```python
from build123d import *

# Parameters (mm, degrees)
SKETCH_W     = 6
SKETCH_H     = 20
PAD_DEPTH    = 4
PAD001_DEPTH = 7
SKETCH002_W  = 2.5
SKETCH002_H  = 20
PAD002_DEPTH = 7
SKETCH003_W  = 4
SKETCH003_H  = 7.068021
PAD003_DEPTH = 9
PAD004_DEPTH = 4
FILLET_R     = 1
FILLET001_R  = 1


with BuildPart() as part:
    # Sketch → Pad (new body)
    with BuildSketch(Plane.XY):
        with Locations((3, -10)):
            Rectangle(SKETCH_W, SKETCH_H)
    extrude(amount=PAD_DEPTH)

    # Sketch001 (on Face6 of Pad) → Pad001 (join)
    with BuildSketch(Plane.XY.offset(4)):
        with BuildLine():
            Line((0, 0), (2.35958, 0))
            ThreePointArc((2.5, -0.14042), (2.458872, -0.041128), (2.35958, 0))
            Line((2.5, -0.14042), (2.5, -0.850163))
            ThreePointArc((2.350164, -0.999998), (2.456114, -0.956113), (2.5, -0.850163))
            Line((2.350164, -0.999998), (1.624627, -0.999998))
            ThreePointArc((1.624627, -0.999998), (1.536498, -1.036503), (1.499994, -1.124632))
            Line((1.499994, -1.124632), (1.499994, -1.858533))
            ThreePointArc((1.499994, -1.858533), (1.541436, -1.958583), (1.641485, -2.000025))
            Line((1.641485, -2.000025), (2.359631, -2.000025))
            ThreePointArc((2.5, -2.140395), (2.458887, -2.041139), (2.359631, -2.000025))
            Line((2.5, -2.140395), (2.5, -2.851653))
            ThreePointArc((2.350363, -3.00129), (2.456173, -2.957463), (2.5, -2.851653))
            Line((2.350363, -3.00129), (1.623935, -3.00129))
            ThreePointArc((1.623935, -3.00129), (1.535246, -3.038027), (1.49851, -3.126716))
            Line((1.49851, -3.126716), (1.49851, -3.86339))
            ThreePointArc((1.49851, -3.86339), (1.54088, -3.965679), (1.643169, -4.008049))
            Line((1.643169, -4.008049), (2.364441, -4.008049))
            ThreePointArc((2.500184, -4.143792), (2.460426, -4.047807), (2.364441, -4.008049))
            Line((2.500184, -4.143792), (2.500184, -4.853508))
            ThreePointArc((2.35038, -5.003311), (2.456307, -4.959435), (2.500184, -4.853508))
            Line((2.35038, -5.003311), (1.6247, -5.003311))
            ThreePointArc((1.6247, -5.003311), (1.536481, -5.039852), (1.49994, -5.128071))
            Line((1.49994, -5.128071), (1.49994, -5.863058))
            ThreePointArc((1.49994, -5.863058), (1.541531, -5.963466), (1.641939, -6.005056))
            Line((1.641939, -6.005056), (2.359895, -6.005056))
            ThreePointArc((2.50033, -6.145492), (2.459198, -6.046189), (2.359895, -6.005056))
            Line((2.50033, -6.145492), (2.50033, -6.855288))
            ThreePointArc((2.350434, -7.005184), (2.456427, -6.961281), (2.50033, -6.855288))
            Line((2.350434, -7.005184), (1.625171, -7.005184))
            ThreePointArc((1.625171, -7.005184), (1.537215, -7.041617), (1.500782, -7.129574))
            Line((1.500782, -7.129574), (1.500782, -7.862621))
            ThreePointArc((1.500782, -7.862621), (1.541938, -7.96198), (1.641297, -8.003136))
            Line((1.641297, -8.003136), (2.356324, -8.003136))
            ThreePointArc((2.500346, -8.147159), (2.458163, -8.04532), (2.356324, -8.003136))
            Line((2.500346, -8.147159), (2.500346, -8.856808))
            ThreePointArc((2.350618, -9.006537), (2.456492, -8.962682), (2.500346, -8.856808))
            Line((2.350618, -9.006537), (1.624599, -9.006537))
            ThreePointArc((1.624599, -9.006537), (1.536168, -9.043166), (1.499538, -9.131597))
            Line((1.499538, -9.131597), (1.499538, -9.865251))
            ThreePointArc((1.499538, -9.865251), (1.541481, -9.966511), (1.642741, -10.008454))
            Line((1.642741, -10.008454), (2.360053, -10.008454))
            ThreePointArc((2.500444, -10.148846), (2.459325, -10.049574), (2.360053, -10.008454))
            Line((2.500444, -10.148846), (2.500444, -10.858493))
            ThreePointArc((2.35072, -11.008218), (2.456591, -10.964364), (2.500444, -10.858493))
            Line((2.35072, -11.008218), (1.634349, -11.008218))
            ThreePointArc((1.634349, -11.008218), (1.545907, -11.044851), (1.509274, -11.133292))
            Line((1.509274, -11.133292), (1.509274, -11.86852))
            ThreePointArc((1.509274, -11.86852), (1.548403, -11.962986), (1.642869, -12.002116))
            Line((1.642869, -12.002116), (2.314983, -12.002116))
            ThreePointArc((2.46352, -12.150526), (2.420007, -12.045539), (2.314983, -12.002116))
            Line((2.46352, -12.150526), (2.46352, -12.860116))
            ThreePointArc((2.350852, -12.972783), (2.43052, -12.939784), (2.46352, -12.860116))
            Line((2.350852, -12.972783), (1.661516, -12.972783))
            ThreePointArc((1.661516, -12.972783), (1.546733, -13.020328), (1.499189, -13.135111))
            Line((1.499189, -13.135111), (1.499189, -13.871471))
            ThreePointArc((1.499189, -13.871471), (1.541454, -13.973508), (1.64349, -14.015773))
            Line((1.64349, -14.015773), (2.364217, -14.015773))
            ThreePointArc((2.500673, -14.152229), (2.460706, -14.05574), (2.364217, -14.015773))
            Line((2.500673, -14.152229), (2.500673, -14.861927))
            ThreePointArc((2.350891, -15.011709), (2.456803, -14.967839), (2.500673, -14.861927))
            Line((2.350891, -15.011709), (1.625116, -15.011709))
            ThreePointArc((1.625116, -15.011709), (1.536839, -15.048275), (1.500273, -15.136553))
            Line((1.500273, -15.136553), (1.500273, -15.871192))
            ThreePointArc((1.500273, -15.871192), (1.541957, -15.971828), (1.642593, -16.013512))
            Line((1.642593, -16.013512), (2.360814, -16.013512))
            ThreePointArc((2.501217, -16.153916), (2.460093, -16.054636), (2.360814, -16.013512))
            Line((2.501217, -16.153916), (2.501217, -16.863601))
            ThreePointArc((2.350997, -17.01382), (2.457218, -16.969822), (2.501217, -16.863601))
            Line((2.350997, -17.01382), (1.625163, -17.01382))
            ThreePointArc((1.625163, -17.01382), (1.537165, -17.05027), (1.500715, -17.138268))
            Line((1.500715, -17.138268), (1.500715, -17.873094))
            ThreePointArc((1.500715, -17.873094), (1.542335, -17.973572), (1.642813, -18.015192))
            Line((1.642813, -18.015192), (2.36048, -18.015192))
            ThreePointArc((2.5009, -18.155612), (2.459772, -18.05632), (2.36048, -18.015192))
            Line((2.5009, -18.155612), (2.5009, -18.865356))
            ThreePointArc((2.351064, -19.015192), (2.457014, -18.971306), (2.5009, -18.865356))
            Line((2.351064, -19.015192), (1.62553, -19.015192))
            ThreePointArc((1.62553, -19.015192), (1.537403, -19.051695), (1.5009, -19.139822))
            Line((1.5009, -19.139822), (1.5009, -20.013354))
            Line((0, -20.013354), (1.5009, -20.013354))
            Line((0, -20.013354), (0, 0))
        make_face()
    extrude(amount=PAD001_DEPTH)

    # Sketch002 (on Face6 of Pad001) → Pad002 (join)
    with BuildSketch(Plane.XY.offset(4)):
        with Locations((4.74459, -10)):
            Rectangle(SKETCH002_W, SKETCH002_H)
    extrude(amount=PAD002_DEPTH)

    # Sketch003 (on Face10 of Pad002) → Pad003 (join)
    with BuildSketch(Plane(origin=(0, 0, 0), x_dir=(0, -1, 0), z_dir=(-1, 0, 0))):
        with Locations((10.057235, 10.469196)):
            Rectangle(SKETCH003_W, SKETCH003_H)
    extrude(amount=PAD003_DEPTH)

    # Sketch004 (on Face95 of Pad003) → Pad004 (join)
    with BuildSketch(Plane(origin=(0, -8.057235, 0), x_dir=(-1, 0, 0), z_dir=(0, 1, 0))):
        Polygon((8.679756, 6.927178), (0, 1.075306), (0, 6.927178), align=None)
    extrude(amount=-PAD004_DEPTH)

    # Fillet
    fillet_edges = [part.edges().sort_by_distance(p)[0] for p in [
        (-9, -8.057235, 10.469196),
    ]]
    fillet(fillet_edges, radius=FILLET_R)

    # Fillet001
    fillet001_edges = [part.edges().sort_by_distance(p)[0] for p in [
        (-9, -12.057235, 10.469196),
    ]]
    fillet(fillet001_edges, radius=FILLET001_R)


solid = part.part
```
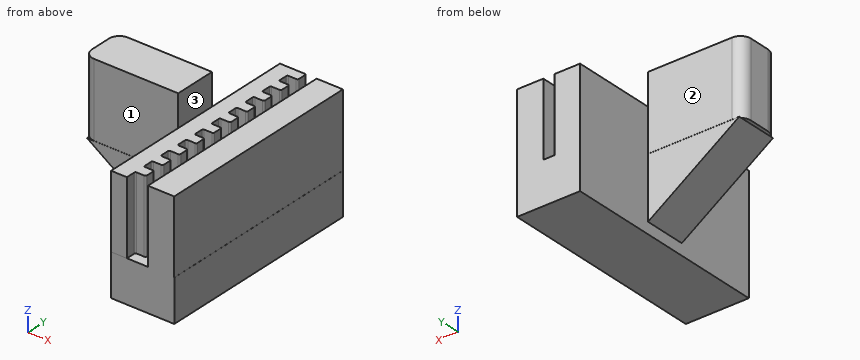
Source: CAD feature listing. Evaluate the final solid. Frame: model axes, mm. Face numbers are marked on the shaded views. A direction names the side the tool comes from. Give positions to 0.01 mm unless a question says otherwise; leave off trailing zeros. Loops run counter-clockwise (first coordinate to the right, second up) from the corner with the lowest first, then second, coordinate; pieces in that order, holes last. Notation, with made-up numbers: M 79.5,38 L 123.5,38 A21 ccw 123.5,75 Z; hole C 60.25,41.25 d1. An arc over 180 degrees is marked long. Put each result on its own line as item: value.
Q1. Section C-C (z = 12.75). Return the cut outline in (x, y).
Response values:
outline: M -9,-11.06 A1 ccw -8,-12.06 L 0,-12.06 L 0,-8.06 L -8,-8.06 A1 ccw -9,-9.06 Z
Q2. Section D-D (x = -1.5). Return the cut outline in (y, z), and give its area (3 significant figures).
Response values:
outline: M -12.06,2.09 L -8.06,2.09 L -8.06,6.93 L -12.06,6.93 Z; M -12.06,6.94 L -8.06,6.94 L -8.06,14 L -12.06,14 Z
area: 47.6 mm²
Q3. Reachability of the marked faces 1, 2 and 3 from +Z, -Z, +X, -X, +Y, -Y: full face, straight path, thin tool, end or side. Return the list, or none.
Response values:
face 1: +Z, -Z, -X, -Y
face 2: +Z, -Z, -X, +Y
face 3: +Z, +X, +Y, -Y
Q4. Pin query (flat end, axial travel): P1, Ø3, axis at x = 4.5, y = -12.5, coming from the +Z side; P2, Ø0.6, axis at y = -1.5, z = 6.5, coming from the +X side; P3, Ø1.5, axis at x = -3.5, z = 11.5, coming from the +Y side. Return the tip coordinate at first contact, or that it passes through.
Response values:
P1: stops at z = 11
P2: stops at x = 5.99
P3: stops at y = -8.06
Q5. Section A-A (x = -3.75). Return the cut outline in (y, z), and give its area (3 significant figures).
Response values:
outline: M -12.06,3.6 L -8.06,3.6 L -8.06,6.93 L -12.06,6.93 Z; M -12.06,6.94 L -8.06,6.94 L -8.06,14 L -12.06,14 Z
area: 41.6 mm²
Q6. Line query: probe 1 along X at (y, z) = (-4.25, 7); probe 2 along X at (y, z) = (-1.25, 9.5); probe 3 along Y at (x, z) = (-6.5, 7.25). Output: solid intervals per line, ascending. Write a range as [from, to].
Response values:
probe 1: x = [0, 2.5], [3.49, 5.99]
probe 2: x = [0, 1.5], [3.49, 5.99]
probe 3: y = [-12.06, -8.06]
